Verification items for this drawing (mm, ordinates from the low corner). Round coordinates to 2 decimals unless told otherwise and drop trailing zeros. Order: outer loops, then holes, each group sorted by start corner. A loop starts at its lowest first (then second) coordinate and runs counter-clockwise, first axis right, second up. Notation, with made-up numbers: (-28.5, -27) -> (18.5, -27) arc R13 ccw to (18.5, -8) -> close; hole circle Ø5 at (54, -8). An arc over 180 degrees is marked (long way). Return JSON: item names as keys, results as strings. Group by question number.
Item 1: Sectioned sample at B-B on z = 1.75. Record the cut outline in (x, y) (3 decimals).
Item 2: Depth check by flat-ended pin: pin 1 Ø3 at (x, y) = (132, 26) entering from +Z; pin 2 Ø1.5 at (y, z) = (6.5, 7) entering from -X; pin 3 Ø1.5 at (x, y) = (101.5, 22.5) entering from -Z; pin 4 Ø2 at (x, y) = (6.35, 25.654) entering from +Z. Enter the tip coordinate at first touch or a pass-through.
Item 3: Sectioned sample at C-C on y = 33.5. Record the cut outline in (x, z).
Item 4: Sectioned sample at D-D on x = 83. Record the cut outline in (y, z), plus the area to 3 significant figures.
Item 5: Sectioned sample at A-A on x = 133.35. Record the cut outline in (y, z), plus the area to 3 significant figures.
Item 6: Scan lines: probe 1 along X at (y, z) = (25.5, 1.5); probe 2 along Y at (x, z) = (133.35, 8.05); probe 3 along Y at (x, z) = (6.35, 5.5). Record each from-to range of solid material in increasing order. Write a range as from..to.
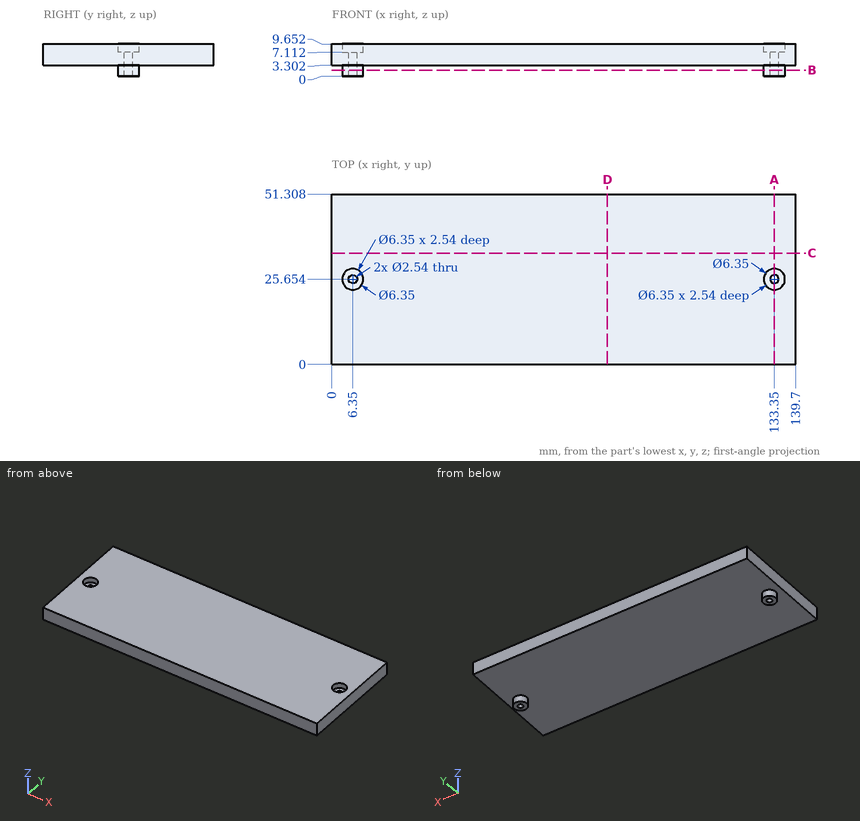
Recorded:
{
 "1": {"outline": "circle Ø6.35 at (6.35, 25.654); circle Ø6.35 at (133.35, 25.654); hole circle Ø2.54 at (6.35, 25.654); hole circle Ø2.54 at (133.35, 25.654)"},
 "2": {"pin 1": "z = 7.11", "pin 2": "x = 0", "pin 3": "z = 3.3", "pin 4": "through"},
 "3": {"outline": "(0, 3.3) -> (139.7, 3.3) -> (139.7, 9.65) -> (0, 9.65) -> close"},
 "4": {"outline": "(0, 3.3) -> (51.31, 3.3) -> (51.31, 9.65) -> (0, 9.65) -> close", "area": "326 mm²"},
 "5": {"outline": "(0, 3.3) -> (22.48, 3.3) -> (22.48, 0) -> (24.38, 0) -> (24.38, 7.11) -> (22.48, 7.11) -> (22.48, 9.65) -> (0, 9.65) -> close; (26.92, 0) -> (28.83, 0) -> (28.83, 3.3) -> (51.31, 3.3) -> (51.31, 9.65) -> (28.83, 9.65) -> (28.83, 7.11) -> (26.92, 7.11) -> close", "area": "313 mm²"},
 "6": {"probe 1": "3.18..5.09, 7.61..9.52, 130.18..132.09, 134.61..136.52", "probe 2": "0..22.48, 28.83..51.31", "probe 3": "0..24.38, 26.92..51.31"}
}
